Geometry: see drawing. Coordinates: mm, zero at the bounding-box minimum. A direction names the side the tool comes from. Round coordinates to 2 decimals unless told otherwise and drop trailing zeros. Write each loop counter-clockwise with the first axis right and the second up, starting at its lowest first coordinate (ties: lowest second). Pieces come first, ordered by that corner, then holes. Notation, with made-up numbers: (15, -1.5) -> (25, -1.5) arc R16 ccw to (25, 24.5) -> close; hole circle Ø2 at (74, 51.5). An arc over 180 degrees is marked (long way). Write item = value, one per line. Start each with the question number.
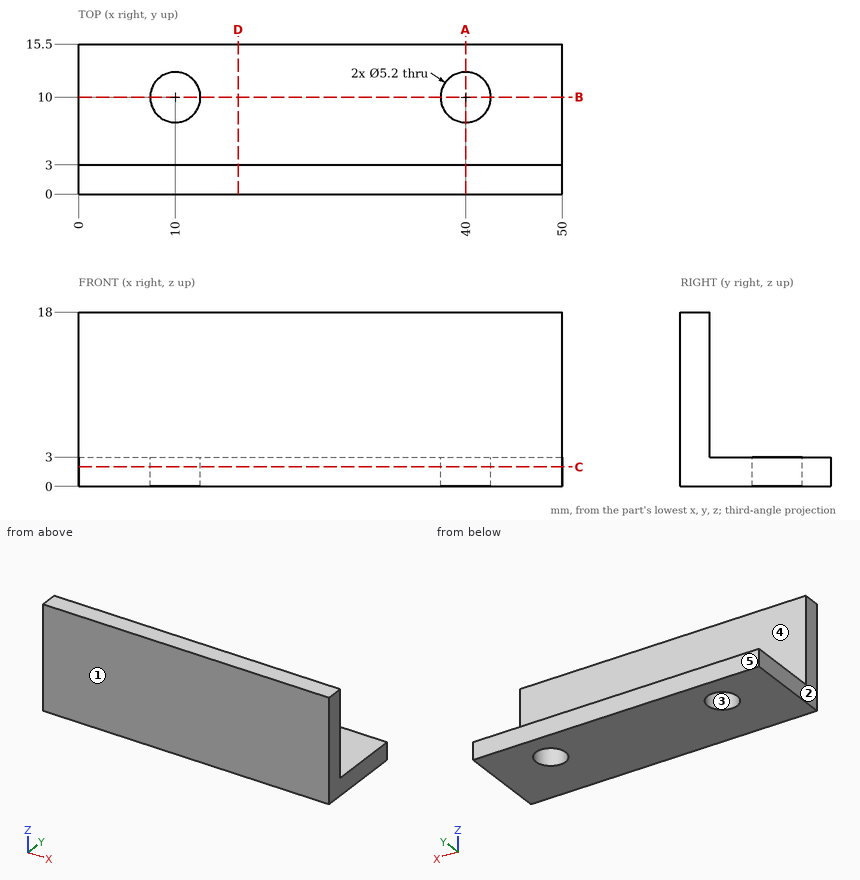
1. Line query: line 1 along Y through (x, z) = (40, 1.8); line 2 along Z through (x, y) = (30.5, 4). Output: solid intervals per line, ascending.
2. Pin query (flat end, axial travel): P1, Ø5, axis at x = 38.5, y = 10, coming from the +Z side. Return the tip coordinate at first contact, or that it passes through.
3. Reachability of the marked faces 4 and 5 from +Z, -Z, +X, -X, +Y, -Y: full face, straight path, thin tool, end or side. Return the list, or none.
4. Section A-A (x = 40). Output: boundary loops of the cut face in (y, z), then the cut area to 3 significant figures.
5. Section D-D (x = 16.5). Output: boundary loops of the cut face in (y, z).
6. Section C-C (z = 2). Output: boundary loops of the cut face in (x, y).
7. Mould query, pull axis Y, two halves, no side actions, for the marked faces 1, 2 and 3. Classes: pulls with the +Y half, pulls with the -Y half, needs draft (parallel to the pull), parting line crosses it, or undercut.
8. Section B-B (y = 10). Output: boundary loops of the cut face in (x, z), then the cut area to 3 significant figures.
Check sheet entries:
q1.line_1 = 0 to 7.4, 12.6 to 15.5
q1.line_2 = 0 to 3
q2.P1 = 3
q3.face_4 = +Z, +X, -X, +Y
q3.face_5 = +Z, -Z, +X, -X, +Y
q4.outline = (0, 0) -> (7.4, 0) -> (7.4, 3) -> (3, 3) -> (3, 18) -> (0, 18) -> close; (12.6, 0) -> (15.5, 0) -> (15.5, 3) -> (12.6, 3) -> close
q4.area = 75.9 mm2
q5.outline = (0, 0) -> (15.5, 0) -> (15.5, 3) -> (3, 3) -> (3, 18) -> (0, 18) -> close
q6.outline = (0, 0) -> (50, 0) -> (50, 15.5) -> (0, 15.5) -> close; hole circle Ø5.2 at (10, 10); hole circle Ø5.2 at (40, 10)
q7.face_1 = pulls with the -Y half
q7.face_2 = needs draft
q7.face_3 = undercut
q8.outline = (0, 0) -> (7.4, 0) -> (7.4, 3) -> (0, 3) -> close; (12.6, 0) -> (37.4, 0) -> (37.4, 3) -> (12.6, 3) -> close; (42.6, 0) -> (50, 0) -> (50, 3) -> (42.6, 3) -> close
q8.area = 119 mm2
